Read the model definition and answer for the solid it produces. Units are mm, in the model's axes. A direction names the side the tool comes from. Coordinates: 2 decimals unless noted, no trailing zeros. Loops run counter-clockwise (first coordinate to the right, second up) from the corner with the lowest first, then second, coordinate; pieces in that order, holes last.
Q1. Which of the six approach directions +Z, -Z, +X, -X, +Y, -Y give full straight-line access (tool end or side, diameter ignored) to faces 1 (the face through (0, 0, 10)), 2 (the face through (0, 0, 20)), 3 (the face through (-1.73, -7.81, 12.6))?
Q2. Section C-C (z = 6.5) is taken. Give the vertices of the cut face in (x, y), then the cut area to 3 significant figures.
Q3. Flat-ended cylindrical pins translate along their axes: P1, Ø3, axis at x = -36, y = -10, coming from the +Z side; P2, Ø12, axis at x = 8, z = -2.5, coming from the -Y side; P3, Ø1.2, axis at x = -0.5, y = 0.5, coming from the -Z side. Find the tip coordinate at first contact, or state that the pin passes through.
Q4. Straight lines are drawn through the part: line 1 (Y direction, x = 0, z = 8); line 2 (Z direction, x = 1, y = 8.5); line 3 (Y direction, x = -5, z = -7.5) (3 decimals). For each, find the intervals that lie inside material, in ascending order.
Q5. Section A-A (y = 0) is taken. Give the vertices of the cut face in (x, z), then the cut area to 3 significant figures.
Q6. Section D-D (z = 18) is taken. Give the vertices of the cut face in (x, y).
from build123d import *

# Parameters (mm, degrees)
SKETCH1_R                = 8
BOSS_EXTRUDE1_DEPTH      = 20
BOSS_EXTRUDE1_DEPTH_BACK = 15
SKETCH2_R                = 45
BOSS_EXTRUDE2_DEPTH      = 5
SKETCH3_R                = 2
CUT_EXTRUDE1_DEPTH       = 10
CUT_EXTRUDE1_DEPTH_BACK  = 15


with BuildPart() as part:
    # Sketch1 → Boss-Extrude1 (new body, two sides)
    with BuildSketch(Plane.XY) as boss_extrude1_sk:
        Circle(SKETCH1_R)
    extrude(amount=BOSS_EXTRUDE1_DEPTH)
    extrude(boss_extrude1_sk.sketch, amount=-BOSS_EXTRUDE1_DEPTH_BACK)

    # Sketch2 → Boss-Extrude2 (add)
    with BuildSketch(Plane.XY):
        Circle(SKETCH2_R)
    extrude(amount=BOSS_EXTRUDE2_DEPTH)

    # Sketch3 → Cut-Extrude1 (cut, two sides)
    with BuildSketch(Plane.XY) as cut_extrude1_sk:
        Circle(SKETCH3_R)
    extrude(amount=CUT_EXTRUDE1_DEPTH, mode=Mode.SUBTRACT)
    extrude(cut_extrude1_sk.sketch, amount=-CUT_EXTRUDE1_DEPTH_BACK, mode=Mode.SUBTRACT)


solid = part.part
Numbers:
1. face 1: -Z
1. face 2: +Z, +X, -X, +Y, -Y
1. face 3: +Z
2. outline: circle Ø16 at (0, 0); hole circle Ø4 at (0, 0)
2. area: 188 mm2
3. P1: stops at z = 5
3. P2: stops at y = -44.93
3. P3: stops at z = 10
4. line 1: y = -8 to -2, 2 to 8
4. line 2: z = 0 to 5
4. line 3: y = -6.245 to 6.245
5. outline: (-45, 0) - (-8, 0) - (-8, -15) - (-2, -15) - (-2, 10) - (2, 10) - (2, -15) - (8, -15) - (8, 0) - (45, 0) - (45, 5) - (8, 5) - (8, 20) - (-8, 20) - (-8, 5) - (-45, 5) - close
5. area: 830 mm2
6. outline: circle Ø16 at (0, 0)
